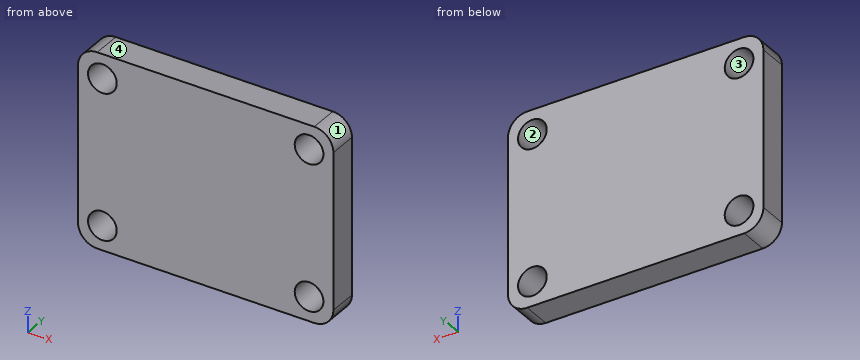
```python
from build123d import *

# Parameters (mm, degrees)
CROQUIS1_W              = 26.67
CROQUIS1_H              = 20.32
SALIENTE_EXTRUIR1_DEPTH = 3
CROQUIS2_R              = 1.5
CORTAR_EXTRUIR1_DEPTH   = 34.662906886
REDONDEO1_R             = 2


with BuildPart() as part:
    # Croquis1 → Saliente-Extruir1 (new body)
    with BuildSketch(Plane(origin=(0, 0, 0), x_dir=(1, 0, 0), z_dir=(0, 1, 0))):
        with Locations((13.335, 10.16)):
            Rectangle(CROQUIS1_W, CROQUIS1_H)
    extrude(amount=SALIENTE_EXTRUIR1_DEPTH)

    # Croquis2 → Cortar-Extruir1 (cut, through all)
    with BuildSketch(Plane(origin=(0, 3, 0), x_dir=(1, 0, 0), z_dir=(0, 1, 0))):
        with Locations(Location((24.13, 2.54, 0), (0, 0, 270))):
            Circle(CROQUIS2_R)
        with Locations(Location((2.54, 2.54, 0), (0, 0, 270))):
            Circle(CROQUIS2_R)
        with Locations(Location((2.54, 17.78, 0), (0, 0, 270))):
            Circle(CROQUIS2_R)
        with Locations(Location((24.13, 17.78, 0), (0, 0, 270))):
            Circle(CROQUIS2_R)
    extrude(amount=-CORTAR_EXTRUIR1_DEPTH, mode=Mode.SUBTRACT)

    # Redondeo1
    redondeo1_edges = [part.edges().sort_by_distance(p)[0] for p in [
        (0, 1.5, -20.32),
        (0, 1.5, 0),
        (26.67, 1.5, 0),
        (26.67, 1.5, -20.32),
    ]]
    fillet(redondeo1_edges, radius=REDONDEO1_R)


solid = part.part
```
Input: part model. Units: mm. Frame: model coordinates. Face numbers are marked on the shaded views. Coordinates: 2 decimals unless noted, no trailing zeros. Write each loop counter-clockwise with the first axis right and the second up, starting at its lowest first coordinate (ties: lowest second). Pieces come first, ordered by that corner, then holes. Notation, with made-up numbers: (8, 37) -> (44, 37) arc R31 ccw to (44, 67) -> close; hole circle Ø2 at (29.25, 68.5). An arc over 180 degrees is marked (long way). Answer as a JSON object with one key per item and string values.
1. Section C-C on y = 0.7. Return the cut outline in (x, z), then the cut area to 3 significant figures.
Result set:
{"outline": "(0, -18.32) arc R2 ccw to (2, -20.32) -> (24.67, -20.32) arc R2 ccw to (26.67, -18.32) -> (26.67, -2) arc R2 ccw to (24.67, 0) -> (2, 0) arc R2 ccw to (0, -2) -> close; hole circle Ø3 at (2.54, -17.78); hole circle Ø3 at (2.54, -2.54); hole circle Ø3 at (24.13, -17.78); hole circle Ø3 at (24.13, -2.54)", "area": "510 mm2"}
2. Section B-B on z = -2.54. Return the cut outline in (x, y), then the cut area to 3 significant figures.
Result set:
{"outline": "(0, 0) -> (1.04, 0) -> (1.04, 3) -> (0, 3) -> close; (4.04, 0) -> (22.63, 0) -> (22.63, 3) -> (4.04, 3) -> close; (25.63, 0) -> (26.67, 0) -> (26.67, 3) -> (25.63, 3) -> close", "area": "62.0 mm2"}
3. Section A-A on x = 2.54. Return the cut outline in (y, z), then the cut area to 3 significant figures.
Result set:
{"outline": "(0, -20.32) -> (3, -20.32) -> (3, -19.28) -> (0, -19.28) -> close; (0, -16.28) -> (3, -16.28) -> (3, -4.04) -> (0, -4.04) -> close; (0, -1.04) -> (3, -1.04) -> (3, 0) -> (0, 0) -> close", "area": "43.0 mm2"}
4. Mould query, pull axis X, two halves, no side actions, for the marked faces 1, 2, 3 and 4. Classes: released by +X, released by -X, zero draft, split by the parting line, or undercut.
Result set:
{"face 1": "released by +X", "face 2": "undercut", "face 3": "undercut", "face 4": "zero draft"}
5. Material intervals for line 1 (X direction, y = 2.75, z = -2.5); line 2 (Z direction, x = 23.25, y = 2.8); line 3 (Z direction, x = 24.5, y = 0.95), sorted ascending. Write a range as from..to.
Result set:
{"line 1": "x = 0..1.04, 4.04..22.63, 25.63..26.67", "line 2": "z = -20.32..-18.99, -16.57..-3.75, -1.33..0", "line 3": "z = -20.32..-19.23, -16.33..-3.99, -1.09..0"}
